from build123d import *

# Parameters (mm, degrees)
SKETCH1_R                               = 10
BOSS_EXTRUDE1_DEPTH                     = 15
CHAMFER1_SIZE                           = 2
CBORE_FOR_M5_HEX_HEAD_BOLT1_D           = 5.5
CBORE_FOR_M5_HEX_HEAD_BOLT1_CBORE_D     = 12.24
CBORE_FOR_M5_HEX_HEAD_BOLT1_CBORE_DEPTH = 5.58


with BuildPart() as part:
    # Sketch1 → Boss-Extrude1 (new body)
    with BuildSketch(Plane.XY):
        Circle(SKETCH1_R)
    extrude(amount=BOSS_EXTRUDE1_DEPTH)

    # Chamfer1
    chamfer1_edges = [part.edges().sort_by_distance(p)[0] for p in [
        (-10, 0, 15),
    ]]
    chamfer(chamfer1_edges, length=CHAMFER1_SIZE)

    # CBORE for M5 Hex Head Bolt1 (through all)
    with Locations(Plane.XY.offset(15)):
        with Locations((0, 0)):
            CounterBoreHole(CBORE_FOR_M5_HEX_HEAD_BOLT1_D / 2, CBORE_FOR_M5_HEX_HEAD_BOLT1_CBORE_D / 2, CBORE_FOR_M5_HEX_HEAD_BOLT1_CBORE_DEPTH)


solid = part.part
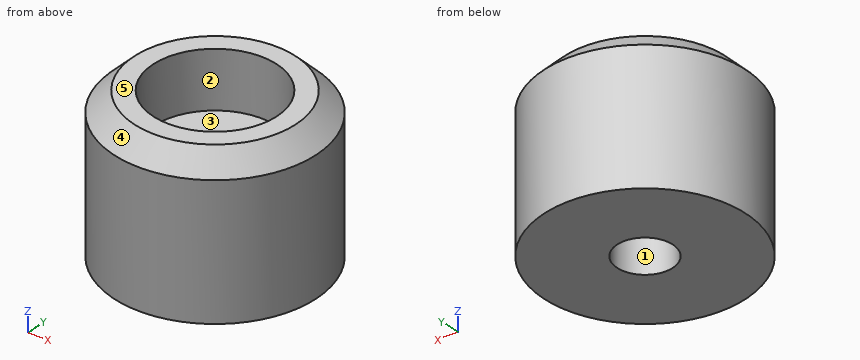
Source: CAD feature listing. Evaluate the final solid. Frame: model axes, mm. Face numbers are marked on the shaded views. A direction names the side the tool comes from. Round coordinates to 2 decimals unless told otherwise and drop trailing zeros. Loops run counter-clockwise (first coordinate to the right, second up) from the corner with the lowest first, then second, coordinate; pieces in that order, holes last.
Q1. Ray query, line 1 (Y direction, x = 0, z = 12.1); line 2 (X direction, y = -1.75, z = 11.75); line 3 (X direction, y = -0.5, z = 13.5). Return the intervals inside material, ascending.
Q2. Section D-D, the plane z = 10.5. Return loops of the section in (x, y), plus the area to 3 significant figures.
Q3. First-contact query: P1, Ø10, axis at x = -0.5, y = -3, coming from the -Z side; P2, Ø1.5, axis at y = 4, z = 5, coming from the +X side; P3, Ø4, axis at y = 4.5, z = 5.5, coming from the -X side. Flat tips, straight axial feed; report the tip coordinate or a pass-through.
Q4. Section C-C, the plane z = 14. Return loops of the section in (x, y).
Q5. Mould query, pull axis Y, two halves, no side actions, for the marked faces 3, 4 and 5. Classes: pulls with the +Y half, pulls with the -Y half, needs draft (parallel to the pull), parting line crosses it, or undercut.
Q6. Section A-A, the plane x = 0. Return loops of the section in (y, z).
Q7. Access query for the marked faces 1 and 2. Directions: +Z, -Z, +X, -X, +Y, -Y. A direction counts if a zero-diameter tool reaches every point of the face in a straight line with its end or side. Return the directions, or none.
Solutions:
1. line 1: y = -10 to -6.12, 6.12 to 10
1. line 2: x = -9.85 to -5.86, 5.86 to 9.85
1. line 3: x = -9.49 to -6.1, 6.1 to 9.49
2. outline: circle Ø20 at (0, 0); hole circle Ø12.24 at (0, 0)
2. area: 196 mm2
3. P1: stops at z = 0
3. P2: stops at x = 9.46
3. P3: stops at x = -9.68
4. outline: circle Ø18 at (0, 0); hole circle Ø12.24 at (0, 0)
5. face 3: undercut
5. face 4: parting line crosses it
5. face 5: needs draft
6. outline: (-10, 0) - (-2.75, 0) - (-2.75, 9.42) - (-6.12, 9.42) - (-6.12, 15) - (-8, 15) - (-10, 13) - close; (2.75, 0) - (10, 0) - (10, 13) - (8, 15) - (6.12, 15) - (6.12, 9.42) - (2.75, 9.42) - close
7. face 1: +Z, -Z
7. face 2: +Z
